Model file for the job. Use its own axes, mm. Face numbers are marked on the shaded views. A direction names the side the tool comes from. Round coordinates to 2 decimals unless told otherwise and drop trailing zeros. Write each loop counter-clockwise with the first axis right and the second up, starting at its lowest first coordinate (ties: lowest second). Pieces come first, ordered by that corner, then holes. Notation, with made-up numbers: (-3.5, 63.5) - (16.5, 63.5) arc R15 cw to (16.5, 82.5) - close; hole circle Ø3 at (86.5, 36). An arc over 180 degrees is marked (long way). One line per item, written item: value.
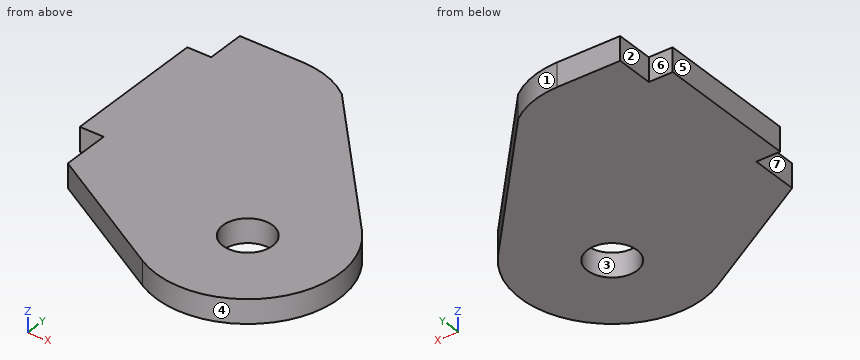
from build123d import *

# Parameters (mm, degrees)
SKETCH1_R           = 3.3
BOSS_EXTRUDE1_DEPTH = 3.175


with BuildPart() as part:
    # Sketch1 → Boss-Extrude1 (new body)
    with BuildSketch(Plane.XY):
        with BuildLine():
            Line((-79.409543338, -48.870574021), (-79.409543338, -29.820574021))
            Line((-79.409543338, -29.820574021), (-76.234543338, -29.820574021))
            Line((-76.234543338, -29.820574021), (-76.234543338, -24.740574021))
            Line((-76.234543338, -24.740574021), (-67.852543338, -24.740574021))
            ThreePointArc((-67.852543338, -24.740574021), (-64.175656813, -25.348124877), (-60.889653149, -27.10618986))
            Line((-60.889653149, -27.10618986), (-43.281292183, -46.938938374))
            ThreePointArc((-43.281292183, -46.938938374), (-43.281292183, -62.612671449), (-58.716906034, -65.334386634))
            Line((-58.716906034, -65.334386634), (-76.234543338, -55.220574021))
            Line((-76.234543338, -55.220574021), (-76.234543338, -48.870574021))
            Line((-76.234543338, -48.870574021), (-79.409543338, -48.870574021))
        make_face()
        with Locations((-52.620906034, -54.775804912)):
            Circle(SKETCH1_R, mode=Mode.SUBTRACT)
    extrude(amount=BOSS_EXTRUDE1_DEPTH)


solid = part.part
1. Band-saw the part on D-D on y = -33. Write the cut outline in (x, z) (3 decimals), plus the area to 3 significant figures.
Report:
outline: (-79.41, 0) - (-55.657, 0) - (-55.657, 3.175) - (-79.41, 3.175) - close
area: 75.4 mm²
2. Drop flat-ended pins along their axis: pin 1 (1.6 mm diameter, centred on y = -51.5, z = 1, fed in from -X); pin 2 (1.5 mm diameter, centred on y = -46.5, z = 2, fed in from +X); pin 3 (1 mm diameter, centred on x = -77.5, z = 1, fed in from +Y). Give the stop position or say it passes through.
Report:
pin 1: x = -76.23
pin 2: x = -43.03
pin 3: y = -29.82
3. Wall check: probe 1 along Y at (x, z) = (-75, 2.85); probe 2 along Y at (x, z) = (-54.5, 0.75); probe 3 along Y at (x, z) = (-68.5, 0.7). Give the ranges that are in metal, low to high. Write a range as [from, to].
Report:
probe 1: [-55.93, -24.74]
probe 2: [-66.82, -57.49], [-52.06, -34.3]
probe 3: [-59.69, -24.74]
4. Mould opens along Y. For the marked faces 1, 2, 3 and 4 say: released by +Y, released by -Y, zero draft, split by the parting line, or undercut.
Report:
face 1: released by +Y
face 2: zero draft
face 3: undercut
face 4: split by the parting line
5. Band-saw the part on A-A on y = -57.5. Write the cut outline in (x, z) (3 decimals), plus the area to 3 significant figures.
Report:
outline: (-72.286, 0) - (-54.483, 0) - (-54.483, 3.175) - (-72.286, 3.175) - close; (-50.758, 0) - (-40.737, 0) - (-40.737, 3.175) - (-50.758, 3.175) - close
area: 88.3 mm²
6. Band-saw the part on C-C on x = -74. Write the cut outline in (y, z) (3 decimals).
Report:
outline: (-56.511, 0) - (-24.741, 0) - (-24.741, 3.175) - (-56.511, 3.175) - close
7. Band-saw the part on B-B on z = 2.2. Write the cut outline in (x, y).
Report:
outline: (-79.41, -48.87) - (-76.23, -48.87) - (-76.23, -55.22) - (-58.72, -65.33) arc R12.19 ccw to (-43.28, -46.94) - (-60.89, -27.11) arc R11.43 ccw to (-67.85, -24.74) - (-76.23, -24.74) - (-76.23, -29.82) - (-79.41, -29.82) - close; hole circle Ø6.6 at (-52.62, -54.78)
8. Tool access for the marked faces 5, 6 and 7: list every direction of +Z, -Z, +X, -X, +Y, -Y with a clear straight run to the whole face (end or side of a thin tool).
Report:
face 5: +Z, -Z, -X, +Y, -Y
face 6: +Z, -Z, -X, +Y
face 7: +Z, -Z, -X, -Y
